Geometry: final body of the model. Coordinates: model frame, mm. Face numbers are marked on the shaded views. A direction names the side the tool comes from. Give positions to 0.01 mm unless a question says otherwise; leave off trailing zeros. Write each loop counter-clockwise with the first axis right and the second up, starting at its lowest first coordinate (ties: lowest second). Pieces come first, ordered by that corner, then holes. Notation, with made-up numbers: M -9.5,61.5 L 23.5,61.5 A23 ccw 23.5,82.5 Z; hole C -31,33 d6. An arc over 180 degrees is marked long. Answer as a JSON object with one key per item and string values.
from build123d import *

# Parameters (mm, degrees)
ESQUISSE1_W             = 50
ESQUISSE1_H             = 44
BOSS_EXTRU_1_DEPTH      = 6
ESQUISSE2_W             = 6
ESQUISSE2_H             = 23.7
ESQUISSE2_W_2           = 17
ESQUISSE2_H_2           = 20.7
ENL_V_MAT_EXTRU_1_DEPTH = 6
ESQUISSE3_W             = 5
ESQUISSE3_H             = 10.7
ENL_V_MAT_EXTRU_2_DEPTH = 6
CONG_1_R                = 4
CONG_2_R                = 1


with BuildPart() as part:
    # Esquisse1 → Boss.-Extru.1 (new body)
    with BuildSketch(Plane.XY):
        with Locations((25, 22)):
            Rectangle(ESQUISSE1_W, ESQUISSE1_H)
    extrude(amount=BOSS_EXTRU_1_DEPTH)

    # Esquisse2 → Enlèv. mat.-Extru.1 (cut)
    with BuildSketch(Plane.XY.offset(6)):
        with Locations((25, 32.15)):
            Rectangle(ESQUISSE2_W, ESQUISSE2_H)
        with Locations((41.5, 33.65)):
            Rectangle(ESQUISSE2_W_2, ESQUISSE2_H_2)
        with Locations((8.5, 33.65)):
            Rectangle(ESQUISSE2_W_2, ESQUISSE2_H_2)
    extrude(amount=-ENL_V_MAT_EXTRU_1_DEPTH, mode=Mode.SUBTRACT)

    # Esquisse3 → Enlèv. mat.-Extru.2 (cut)
    with BuildSketch(Plane.XY.offset(6)):
        with Locations((19.5, 38.65)):
            Rectangle(ESQUISSE3_W, ESQUISSE3_H)
        with Locations((30.5, 38.65)):
            Rectangle(ESQUISSE3_W, ESQUISSE3_H)
    extrude(amount=-ENL_V_MAT_EXTRU_2_DEPTH, mode=Mode.SUBTRACT)

    # Congé1
    cong_1_edges = [part.edges().sort_by_distance(p)[0] for p in [
        (50, 23.3, 3),
        (0, 23.3, 3),
        (50, 0, 3),
        (0, 0, 3),
    ]]
    fillet(cong_1_edges, radius=CONG_1_R)

    # Congé2
    cong_2_edges = [part.edges().sort_by_distance(p)[0] for p in [
        (33, 23.3, 3),
        (17, 23.3, 3),
        (17, 33.3, 3),
        (22, 33.3, 3),
        (28, 33.3, 3),
        (33, 33.3, 3),
    ]]
    fillet(cong_2_edges, radius=CONG_2_R)


solid = part.part
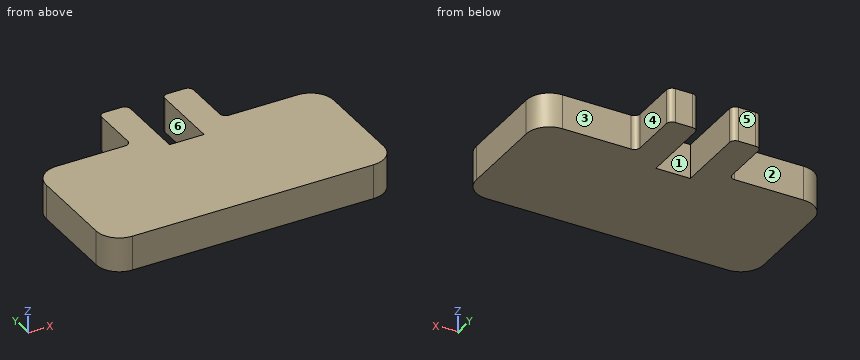
1) Set-up query: the marked faces 1, 2 and 3. Return all of +Z, -Z, +X, -X, +Y, -Y with unobstructed straight access to the full face (end or side cutting, diameter ignored); none if empty.
Geometry check:
{"face 1": "+Z, -Z, +Y", "face 2": "+Z, -Z, -X, +Y", "face 3": "+Z, -Z, +X, +Y"}
2) Cut plane B-B on z = 4.8. Return loops of the section in (x, y).
Geometry check:
{"outline": "M 0,4 A4 ccw 4,0 L 46,0 A4 ccw 50,4 L 50,19.3 A4 ccw 46,23.3 L 34,23.3 A1 cw 33,24.3 L 33,32.3 A1 ccw 32,33.3 L 29,33.3 A1 ccw 28,32.3 L 28,20.3 L 22,20.3 L 22,32.3 A1 ccw 21,33.3 L 18,33.3 A1 ccw 17,32.3 L 17,24.3 A1 cw 16,23.3 L 4,23.3 A4 ccw 0,19.3 Z"}
3) Cut plane C-C on y = 21.5. Return loops of the section in (x, z).
Geometry check:
{"outline": "M 0.66,0 L 22,0 L 22,6 L 0.66,6 Z; M 28,0 L 49.34,0 L 49.34,6 L 28,6 Z"}
4) Cut plane A-A on y = 31. Return loops of the section in (x, z), and give its area (3 significant figures).
Geometry check:
{"outline": "M 17,0 L 22,0 L 22,6 L 17,6 Z; M 28,0 L 33,0 L 33,6 L 28,6 Z", "area": "60.0 mm2"}
5) Contact query for flat-ended pins moving along their axis: P1, Ø1.8, axis at x = 38.5, z = 4, coming from the +Y side; P2, Ø3, axis at x = 25.5, z = 2, coming from the +Y side; P3, Ø3, axis at y = 29.5, z = 2.5, coming from the -X side. Output: stop coordinate, or through.
Geometry check:
{"P1": "stops at y = 23.3", "P2": "stops at y = 20.3", "P3": "stops at x = 17"}
6) Cut plane D-D on x = 14. Return loops of the section in (y, z), and give its area (3 significant figures).
Geometry check:
{"outline": "M 0,0 L 23.3,0 L 23.3,6 L 0,6 Z", "area": "140 mm2"}
7) Pull-direction query (X, two-part tool) for the marked faces 4, 5 and 6; classes: pulls with the +X half, pulls with the -X half, needs draft (parallel to the pull), parting line crosses it, or undercut.
Geometry check:
{"face 4": "pulls with the +X half", "face 5": "needs draft", "face 6": "undercut"}
8) Line query: line 1 (X direction, y = 28, z = 5.5); line 2 (X direction, y = 23.5, z = 1.4); line 3 (Y direction, x = 25, z = 4.05). Output: solid intervals per line, ascending. Write a range as from..to.
Geometry check:
{"line 1": "x = 17..22, 28..33", "line 2": "x = 16.6..22, 28..33.4", "line 3": "y = 0..20.3"}
